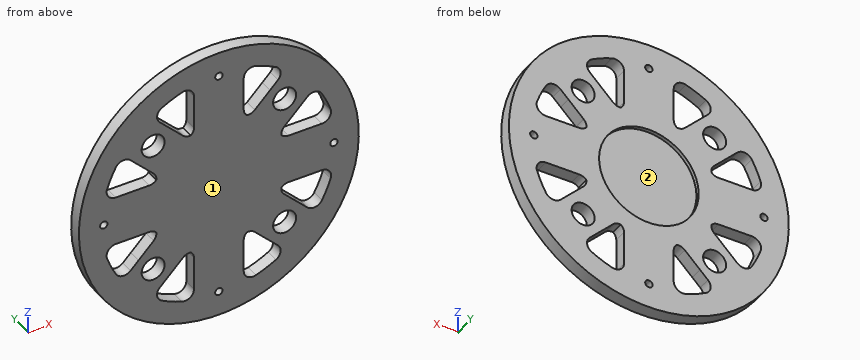
from build123d import *

# Parameters (mm, degrees)
SKETCH1_R           = 76
SKETCH1_R_2         = 27.051
SKETCH1_R_3         = 2
BOSS_EXTRUDE1_DEPTH = 7
SKETCH3_R           = 27.051
BOSS_EXTRUDE2_DEPTH = 5
SKETCH4_R           = 6.25
CUT_EXTRUDE1_DEPTH  = 10
FILLET1_R           = 5


with BuildPart() as part:
    # Sketch1 → Boss-Extrude1 (new body)
    with BuildSketch(Plane(origin=(0, 0, 0), x_dir=(1, 0, 0), z_dir=(0, 1, 0))):
        with Locations(Location((0, 0, 0), (0, 0, 270))):
            Circle(SKETCH1_R)
        with Locations(Location((0, 0, 0), (0, 0, 270))):
            Circle(SKETCH1_R_2, mode=Mode.SUBTRACT)
        with Locations(Location((0, 62.5, 0), (0, 0, 270))):
            Circle(SKETCH1_R_3, mode=Mode.SUBTRACT)
        with Locations(Location((62.5, 0, 0), (0, 0, 270))):
            Circle(SKETCH1_R_3, mode=Mode.SUBTRACT)
        with Locations(Location((0, -62.5, 0), (0, 0, 270))):
            Circle(SKETCH1_R_3, mode=Mode.SUBTRACT)
        with Locations(Location((-62.5, 0, 0), (0, 0, 270))):
            Circle(SKETCH1_R_3, mode=Mode.SUBTRACT)
    extrude(amount=BOSS_EXTRUDE1_DEPTH)

    # Sketch3 → Boss-Extrude2 (add)
    with BuildSketch(Plane.XZ):
        with Locations(Location((0, 0, 0), (0, 0, 270))):
            Circle(SKETCH3_R)
    extrude(amount=-BOSS_EXTRUDE2_DEPTH)

    # Sketch4 → Cut-Extrude1 (cut)
    with BuildSketch(Plane(origin=(0, 7, 0), x_dir=(1, 0, 0), z_dir=(0, 1, 0))):
        with BuildLine():
            Line((27.751246841, -43.661149418), (17.007161012, -32.917063589))
            ThreePointArc((17.007161012, -32.917063589), (15.274204293, -33.756114768), (13.5, -34.504008477))
            Line((13.5, -34.504008477), (13.5, -62.5))
            ThreePointArc((13.5, -62.5), (25.524772494, -58.625813335), (36.553123822, -52.463026398))
            Line((36.553123822, -52.463026398), (27.751246841, -43.661149418))
        make_face()
        with BuildLine():
            Line((62.5, -13.5), (34.504008477, -13.5))
            ThreePointArc((34.504008477, -13.5), (33.756114768, -15.274204293), (32.917063589, -17.007161012))
            Line((32.917063589, -17.007161012), (43.66114941, -27.751246833))
            Line((43.66114941, -27.751246833), (52.463026398, -36.553123822))
            ThreePointArc((52.463026398, -36.553123822), (58.625813335, -25.524772494), (62.5, -13.5))
        make_face()
        with BuildLine():
            ThreePointArc((-13.5, -34.504008477), (-15.274204293, -33.756114768), (-17.007161012, -32.917063589))
            Line((-17.007161012, -32.917063589), (-27.751246874, -43.66114945))
            Line((-27.751246874, -43.66114945), (-36.553123822, -52.463026398))
            ThreePointArc((-36.553123822, -52.463026398), (-25.524772494, -58.625813335), (-13.5, -62.5))
            Line((-13.5, -62.5), (-13.5, -34.504008477))
        make_face()
        with BuildLine():
            ThreePointArc((-32.917063589, -17.007161012), (-33.756114768, -15.274204293), (-34.504008477, -13.5))
            Line((-34.504008477, -13.5), (-62.5, -13.5))
            ThreePointArc((-62.5, -13.5), (-58.625813335, -25.524772494), (-52.463026398, -36.553123822))
            Line((-52.463026398, -36.553123822), (-43.661149471, -27.751246894))
            Line((-43.661149471, -27.751246894), (-32.917063589, -17.007161012))
        make_face()
        with BuildLine():
            ThreePointArc((-34.504008477, 13.5), (-33.756114768, 15.274204293), (-32.917063589, 17.007161012))
            Line((-32.917063589, 17.007161012), (-43.66114943, 27.751246854))
            Line((-43.66114943, 27.751246854), (-52.463026398, 36.553123822))
            ThreePointArc((-52.463026398, 36.553123822), (-58.625813335, 25.524772494), (-62.5, 13.5))
            Line((-62.5, 13.5), (-34.504008477, 13.5))
        make_face()
        with BuildLine():
            ThreePointArc((-17.007161012, 32.917063589), (-15.274204293, 33.756114768), (-13.5, 34.504008477))
            Line((-13.5, 34.504008477), (-13.5, 62.5))
            ThreePointArc((-13.5, 62.5), (-25.524772494, 58.625813335), (-36.553123822, 52.463026398))
            Line((-36.553123822, 52.463026398), (-27.751246874, 43.66114945))
            Line((-27.751246874, 43.66114945), (-17.007161012, 32.917063589))
        make_face()
        with BuildLine():
            ThreePointArc((36.553123822, 52.463026398), (25.524772494, 58.625813335), (13.5, 62.5))
            Line((13.5, 62.5), (13.5, 34.504008477))
            ThreePointArc((13.5, 34.504008477), (15.274204293, 33.756114768), (17.007161012, 32.917063589))
            Line((17.007161012, 32.917063589), (27.751246906, 43.661149483))
            Line((27.751246906, 43.661149483), (36.553123822, 52.463026398))
        make_face()
        with BuildLine():
            ThreePointArc((62.5, 13.5), (58.625813335, 25.524772494), (52.463026398, 36.553123822))
            Line((52.463026398, 36.553123822), (43.66114945, 27.751246874))
            Line((43.66114945, 27.751246874), (32.917063589, 17.007161012))
            ThreePointArc((32.917063589, 17.007161012), (33.756114768, 15.274204293), (34.504008477, 13.5))
            Line((34.504008477, 13.5), (62.5, 13.5))
        make_face()
        with Locations(Location((35.706198162, 35.706198162, 0), (0, 0, 270))):
            Circle(SKETCH4_R)
        with Locations(Location((35.706198162, -35.706198162, 0), (0, 0, 270))):
            Circle(SKETCH4_R)
        with Locations(Location((-35.706198162, -35.706198162, 0), (0, 0, 270))):
            Circle(SKETCH4_R)
        with Locations(Location((-35.706198162, 35.706198162, 0), (0, 0, 270))):
            Circle(SKETCH4_R)
    extrude(amount=-CUT_EXTRUDE1_DEPTH, mode=Mode.SUBTRACT)

    # Fillet1
    # the kernel refuses this fillet: 5 mm, written as the material it adds along each edge
    with BuildSketch(Plane(origin=(34.504008477, 7, 13.5), x_dir=(1, 0, 0), z_dir=(0, -1, 0)), Plane(origin=(13.5, 7, -34.504008477), x_dir=(0, 0, -1), z_dir=(0, -1, 0)), Plane(origin=(-34.504008477, 7, -13.5), x_dir=(-1, 0, 0), z_dir=(0, -1, 0)), Plane(origin=(-13.5, 7, 34.504008477), x_dir=(0, 0, 1), z_dir=(0, -1, 0))) as fillet1_piece_1:
        with BuildLine():
            CenterArc((3.258891319, 5), FILLET1_R, 206.100178987, 63.899821013)
            ThreePointArc((-1.231239688, 2.800290124), (-0.586707725, 1.412857227), (0, 0))
            Line((0, 0), (3.258891319, 0))
        make_face()
    extrude(amount=7)
    with BuildSketch(Plane(origin=(62.5, 7, 13.5), x_dir=(-1, 0, 0), z_dir=(0, -1, 0))) as fillet1_piece_2:
        with BuildLine():
            CenterArc((6.537189081, -5), FILLET1_R, 90, 108.2926811)
            ThreePointArc((1.789861186, -6.569355874), (0.807426008, -3.308519097), (0, 0))
            Line((0, 0), (6.537189081, 0))
        make_face()
    extrude(amount=7)
    with BuildSketch(Plane(origin=(52.463026398, 7, 36.553123822), x_dir=(-0.7071067811865521, 0, -0.707106781186543), z_dir=(0, -1, 0)), Plane(origin=(-36.553123822, 7, 52.463026398), x_dir=(0.7071067811865515, 0, -0.7071067811865436), z_dir=(0, -1, 0))) as fillet1_piece_3:
        with BuildLine():
            CenterArc((6.286852353, 5), FILLET1_R, 163.996405934, 106.003594066)
            ThreePointArc((1.480630334, 6.378488268), (0.658610883, 3.208210045), (0, 0))
            Line((0, 0), (6.286852353, 0))
        make_face()
    extrude(amount=7)
    with BuildSketch(Plane(origin=(32.917063589, 7, 17.007161012), x_dir=(0.4193809358930841, 0, -0.907810349472532), z_dir=(0, -1, 0)), Plane(origin=(17.007161012, 7, -32.917063589), x_dir=(-0.9078103494725283, 0, -0.41938093589309267), z_dir=(0, -1, 0)), Plane(origin=(-32.917063589, 7, -17.007161012), x_dir=(-0.4193809358930852, 0, 0.9078103494725317), z_dir=(0, -1, 0))) as fillet1_piece_4:
        with BuildLine():
            CenterArc((3.489548398, 4.995132399), FILLET1_R, 200.204490443, 67.267112024)
            Line((-1.202781391, 3.268273647), (0, 0))
            ThreePointArc((0, 0), (1.634487847, 0.036069898), (3.268975694, 0))
        make_face()
    extrude(amount=7)
    with BuildSketch(Plane(origin=(32.917063589, 7, -17.007161012), x_dir=(0.7071067811865526, 0, -0.7071067811865425), z_dir=(0, -1, 0)), Plane(origin=(-17.007161012, 7, -32.917063589), x_dir=(-0.7071067811865506, 0, -0.7071067811865445), z_dir=(0, -1, 0)), Plane(origin=(-32.917063589, 7, 17.007161012), x_dir=(-0.7071067811865506, 0, 0.7071067811865445), z_dir=(0, -1, 0)), Plane(origin=(17.007161012, 7, 32.917063589), x_dir=(0.7071067811865501, 0, 0.707106781186545), z_dir=(0, -1, 0))) as fillet1_piece_5:
        with BuildLine():
            CenterArc((3.482570273, 5), FILLET1_R, 202.732887976, 67.267112024)
            ThreePointArc((-1.129011858, 3.067822406), (-0.530655558, 1.546368727), (0, 0))
            Line((0, 0), (3.482570273, 0))
        make_face()
    extrude(amount=7)
    with BuildSketch(Plane(origin=(34.504008477, 7, -13.5), x_dir=(1, 0, 0), z_dir=(0, -1, 0))) as fillet1_piece_6:
        with BuildLine():
            CenterArc((3.258891319, -5), FILLET1_R, 90, 63.899821013)
            ThreePointArc((-1.231239688, -2.800290124), (-0.586707725, -1.412857227), (0, 0))
            Line((0, 0), (3.258891319, 0))
        make_face()
    extrude(amount=7)
    with BuildSketch(Plane(origin=(62.5, 7, -13.5), x_dir=(-1, 0, 0), z_dir=(0, -1, 0)), Plane(origin=(-13.5, 7, -62.5), x_dir=(0, 0, 1), z_dir=(0, -1, 0)), Plane(origin=(-62.5, 7, 13.5), x_dir=(1, 0, 0), z_dir=(0, -1, 0)), Plane(origin=(13.5, 7, 62.5), x_dir=(0, 0, -1), z_dir=(0, -1, 0))) as fillet1_piece_7:
        with BuildLine():
            CenterArc((6.537189081, 5), FILLET1_R, 161.7073189, 108.2926811)
            ThreePointArc((1.789861186, 6.569355874), (0.807426008, 3.308519097), (0, 0))
            Line((0, 0), (6.537189081, 0))
        make_face()
    extrude(amount=7)
    with BuildSketch(Plane(origin=(52.463026398, 7, -36.553123822), x_dir=(0.5289042688396526, 0, 0.848681491728901), z_dir=(0, -1, 0))) as fillet1_piece_8:
        with BuildLine():
            CenterArc((6.292063112, 4.993441128), FILLET1_R, 166.931450544, 106.003594066)
            Line((1.421561948, 6.124024341), (0, 0))
            ThreePointArc((0, 0), (3.274041034, -0.08387667), (6.548082068, 0))
        make_face()
    extrude(amount=7)
    with BuildSketch(Plane(origin=(36.553123822, 7, -52.463026398), x_dir=(-0.8486814917288963, 0, -0.52890426883966), z_dir=(0, -1, 0)), Plane(origin=(-52.463026398, 7, -36.553123822), x_dir=(-0.5289042688396536, 0, 0.8486814917289003), z_dir=(0, -1, 0))) as fillet1_piece_9:
        with BuildLine():
            CenterArc((6.292063112, -4.993441128), FILLET1_R, 87.06495539, 106.003594066)
            Line((1.421561948, -6.124024341), (0, 0))
            ThreePointArc((0, 0), (3.274041034, 0.08387667), (6.548082068, 0))
        make_face()
    extrude(amount=7)
    with BuildSketch(Plane(origin=(13.5, 7, -62.5), x_dir=(0.9648302017860143, 0, 0.26287388938720957), z_dir=(0, -1, 0)), Plane(origin=(-62.5, 7, -13.5), x_dir=(0.2628738893872084, 0, -0.9648302017860146), z_dir=(0, -1, 0)), Plane(origin=(-13.5, 7, 62.5), x_dir=(-0.9648302017860145, 0, -0.26287388938720885), z_dir=(0, -1, 0))) as fillet1_piece_10:
        with BuildLine():
            CenterArc((6.542607328, 4.992908013), FILLET1_R, 164.759342849, 108.2926811)
            Line((1.718456319, 6.30727746), (0, 0))
            ThreePointArc((0, 0), (3.404410363, -0.090694285), (6.808820725, 0))
        make_face()
    extrude(amount=7)
    with BuildSketch(Plane(origin=(-36.553123822, 7, -52.463026398), x_dir=(0.707106781186552, 0, 0.7071067811865429), z_dir=(0, -1, 0)), Plane(origin=(-52.463026398, 7, 36.553123822), x_dir=(0.7071067811865515, 0, -0.7071067811865436), z_dir=(0, -1, 0)), Plane(origin=(36.553123822, 7, 52.463026398), x_dir=(-0.7071067811865527, 0, -0.7071067811865425), z_dir=(0, -1, 0))) as fillet1_piece_11:
        with BuildLine():
            CenterArc((6.286852353, -5), FILLET1_R, 90, 106.003594066)
            ThreePointArc((1.480630334, -6.378488268), (0.658610883, -3.208210045), (0, 0))
            Line((0, 0), (6.286852353, 0))
        make_face()
    extrude(amount=7)
    with BuildSketch(Plane(origin=(-13.5, 7, -34.504008477), x_dir=(-0.9154220062230544, 0, 0.4024954043496127), z_dir=(0, -1, 0)), Plane(origin=(-34.504008477, 7, 13.5), x_dir=(0.4024954043496181, 0, 0.915422006223052), z_dir=(0, -1, 0)), Plane(origin=(13.5, 7, 34.504008477), x_dir=(0.915422006223051, 0, -0.40249540434962), z_dir=(0, -1, 0))) as fillet1_piece_12:
        with BuildLine():
            CenterArc((3.265421252, 4.995737851), FILLET1_R, 203.734271223, 63.899821013)
            Line((-1.311688779, 2.983260829), (0, 0))
            ThreePointArc((0, 0), (1.52950776, 0.031583378), (3.059015519, 0))
        make_face()
    extrude(amount=7)
    with BuildSketch(Plane(origin=(-17.007161012, 7, 32.917063589), x_dir=(-0.7071067811865496, 0, 0.7071067811865455), z_dir=(0, -1, 0))) as fillet1_piece_13:
        with BuildLine():
            CenterArc((3.482570273, -5), FILLET1_R, 90, 67.267112024)
            ThreePointArc((-1.129011858, -3.067822406), (-0.530655558, -1.546368727), (0, 0))
            Line((0, 0), (3.482570273, 0))
        make_face()
    extrude(amount=7)


solid = part.part
Here's how the part is built. I have some questions about the finished solid (model axes, mm). Face numbers are marked on the shaded views. A direction names the side the tool comes from. Coordinates: 2 decimals unless noted, no trailing zeros. Loops run counter-clockwise (first coordinate to the right, second up) from the corner with the lowest first, then second, coordinate; pieces in that order, holes last.
1. For the marked faces 1 and 2, which set-ups out of +Z, -Z, +X, -X, +Y, -Y let a thin tool reach every point of the face, with its end or its side?
2. Imagine slicing it at D-D, the plane z = -67. Please give me the cut outline in (x, y), and give its area (3 significant figures).
3. Imagine slicing it at A-A, the plane z = 0. Please give me the cut outline in (x, y).
4. Imagine slicing it at B-B, the plane x = 0. Please give me the cut outline in (y, z).
5. Imagine slicing it at C-C, the plane y = 1.75. Count the separate pieces of the cut face and the enclosed holes in it, and give its area (3 significant figures).
6. I need wall thicknesses on L1, parallel to X at y = 4.25, z = 0; L2, parallel to X at y = 4.75, z = -17.5; L3, parallel to Z at x = 29, y = 2.25. Which ranges of each line are inside material? Lowest first, please.
7. For P1, Ø1, axis at y = 4.5, z = 11.5, coming from the -X side; P2, Ø2, axis at y = 3, z = 47, coming from the -X side; P3, Ø3.5, axis at y = 5, z = 48, coming from the +X side, each with a flat end and sliding along its axis, tell me the tip position at first contact or that it passes through.
Taken from the geometry:
1. face 1: +Z, -Z, +X, -X, -Y
1. face 2: +Y
2. outline: (-35.87, 0) - (35.87, 0) - (35.87, 7) - (-35.87, 7) - close
2. area: 502 mm2
3. outline: (-76, 0) - (-64.5, 0) - (-64.5, 7) - (-76, 7) - close; (-60.5, 0) - (60.5, 0) - (60.5, 7) - (27.05, 7) - (27.05, 5) - (-27.05, 5) - (-27.05, 7) - (-60.5, 7) - close; (64.5, 0) - (76, 0) - (76, 7) - (64.5, 7) - close
4. outline: (0, -76) - (7, -76) - (7, -64.5) - (0, -64.5) - close; (0, -60.5) - (7, -60.5) - (7, -27.05) - (5, -27.05) - (5, 27.05) - (7, 27.05) - (7, 60.5) - (0, 60.5) - close; (0, 64.5) - (7, 64.5) - (7, 76) - (0, 76) - close
5. separate pieces: 1
5. enclosed holes: 16
5. area: 14,600 mm2
6. L1: x = -76 to -64.5, -60.5 to 60.5, 64.5 to 76
6. L2: x = -73.96 to -60.86, -34.17 to 34.17, 60.86 to 73.96
6. L3: z = -70.25 to -56.99, -44.91 to 44.91, 56.99 to 70.25
7. P1: stops at x = -75.2
7. P2: stops at x = -60.5
7. P3: stops at x = 60.31
